Geometry: final body of the model. Coordinates: model frame, mm. Give positions to 0.01 mm unless a question says otherwise; leave off trailing zeros. Write each loop counter-clockwise with the first axis right and the second up, starting at its lowest first coordinate (ties: lowest second). Pieces come first, ordered by that corner, then holes. Notation, with made-up numbers: (-7.75, -30.5) -> (47.25, -30.5) arc R30 cw to (47.25, 7.5) -> close; hole circle Ø8 at (6, 69.5). An arc over 180 degrees is marked (long way). Answer as a JSON object with one key per item and string values. Group by question number.
(1) Contact query for a flat-ended pin moving along its axis: pin 1 Ø2.5 at (x, y) = (-90, 17.5) entering from +Z. Output: stop coordinate, or through.
(2) Material intervals for probe 1 along Y at (x, z) = (90, 1.2); probe 2 along Y at (x, z) = (14.25, 2.45); probe 3 along X at (y, z) = (26, 2.15), sorted ascending.
(3) Section query A-A on y = -5.5. Output: boundary loops of the cut face in (x, z), plus the area to 3 significant figures.
from build123d import *

# Parameters (mm, degrees)
ESBO_O1_W                = 200
ESBO_O1_H                = 250
ESBO_O1_R                = 1.8
ESBO_O1_R_2              = 2
RESSALTO_EXTRUS_O1_DEPTH = 3


with BuildPart() as part:
    # Esboço1 → Ressalto-extrusão1 (new body)
    with BuildSketch(Plane.XY):
        Rectangle(ESBO_O1_W, ESBO_O1_H)
        with Locations((-14.25, 25)):
            Circle(ESBO_O1_R, mode=Mode.SUBTRACT)
        with Locations((14.25, 25)):
            Circle(ESBO_O1_R, mode=Mode.SUBTRACT)
        with Locations((14.25, 2.5)):
            Circle(ESBO_O1_R, mode=Mode.SUBTRACT)
        with Locations((-14.25, 2.5)):
            Circle(ESBO_O1_R, mode=Mode.SUBTRACT)
        with Locations((-90, -92.5)):
            Circle(ESBO_O1_R_2, mode=Mode.SUBTRACT)
        with Locations((-90, 17.5)):
            Circle(ESBO_O1_R_2, mode=Mode.SUBTRACT)
        with Locations((90, 17.5)):
            Circle(ESBO_O1_R_2, mode=Mode.SUBTRACT)
        with Locations((90, -92.5)):
            Circle(ESBO_O1_R_2, mode=Mode.SUBTRACT)
        with BuildLine():
            Line((-63.2, 5), (-63.2, -65))
            ThreePointArc((-63.2, -65), (-65, -66.8), (-66.8, -65))
            Line((-66.8, -65), (-66.8, 5))
            ThreePointArc((-66.8, 5), (-65, 6.8), (-63.2, 5))
        make_face(mode=Mode.SUBTRACT)
    extrude(amount=RESSALTO_EXTRUS_O1_DEPTH)


solid = part.part
Answer list:
{
 "1": {"pin 1": "through"},
 "2": {"probe 1": "-125 to -94.5, -90.5 to 15.5, 19.5 to 125", "probe 2": "-125 to 0.7, 4.3 to 23.2, 26.8 to 125", "probe 3": "-100 to -15.75, -12.75 to 12.75, 15.75 to 100"},
 "3": {"outline": "(-100, 0) -> (-66.8, 0) -> (-66.8, 3) -> (-100, 3) -> close; (-63.2, 0) -> (100, 0) -> (100, 3) -> (-63.2, 3) -> close", "area": "589 mm2"}
}
